Geometry check sheet. Reference: the model listing, model coordinates, mm. Face numbers are marked on the shaded views. Coordinates: 2 decimals unless noted, no trailing zeros. Write each loop counter-clockwise with the first axis right and the second up, starting at its lowest first coordinate (ties: lowest second). Pieces come first, ordered by that corner, then holes. Notation, with made-up numbers: (17, 44.25) -> (36, 44.25) arc R12 cw to (36, 48.25) -> close; hole circle Ø6 at (39.5, 71.25). An arc over 180 degrees is marked (long way). Answer in a Markdown table with one row per item. Add a question column.
1. Depth check by flat-ended pin: P1, Ø0.5, axis at x = 31.5, z = -72.5, coming from the +Y side; P2, Ø2.5, axis at x = -20.5, z = -49, coming from the +Y side; P3, Ø16.5, axis at x = 9, y = 7.5, coming from the -Z side. Enter the tip coordinate at first touch or a pass-through.
2. Mould release check, pull along Y, two halves, no side actions. Record for the marked faces 1, 2, 3 and 4: pulls with the +Y half, pulls with the -Y half, needs draft (parallel to the pull), parting line crosses it, or undercut.
3. Scan lines: L1, parallel to Y at x = 25, z = -16; L2, parallel to X at y = -13, z = -5.5; L3, parallel to X at y = 9.5, z = -63. Record each from-to range of solid material in increasing order. Write a range as from..to.
4. Cross-section at B-B on x = -20.5. Give the number of separate pieces and of enclosed holes in the cut face, and give its area (3 significant figures).
5. Cross-section at D-D on z = -66. Record the cut outline in (x, y).
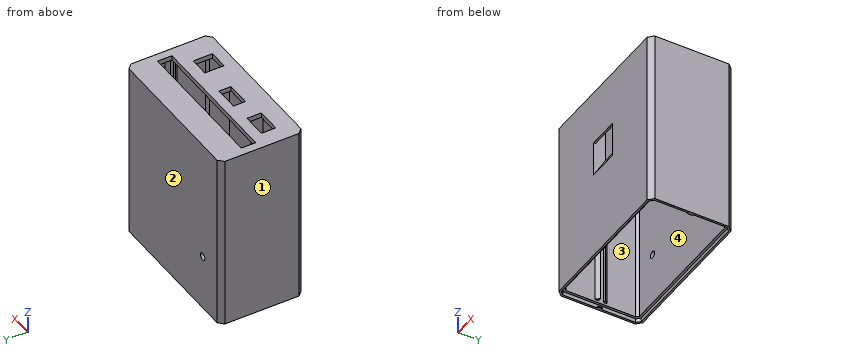
```python
from build123d import *
from OCP.BRepFilletAPI import BRepFilletAPI_MakeChamfer

# Parameters (mm, degrees)
CROQUIS1_W              = 3.5
CROQUIS1_H              = 6
CROQUIS1_W_2            = 10
CROQUIS1_H_2            = 5
CROQUIS1_W_3            = 8
CROQUIS1_H_3            = 8
SALIENTE_EXTRUIR1_DEPTH = 2
CROQUIS2_W              = 65
CROQUIS2_H              = 35
CROQUIS2_W_2            = 61
CROQUIS2_H_2            = 31
SALIENTE_EXTRUIR2_DEPTH = 71
SALIENTE_EXTRUIR3_DEPTH = 70
CORTAR_EXTRUIR2_REACH   = 87.57
CROQUIS9_R              = 1.5
CHAFL_N3_SIZE           = 2
CHAFL_N2_SIZE           = 1
BOSS_EXTRUDE1_DEPTH     = 1.5
CHAMFER1_SIZE           = 0.1
CHAMFER1_SIZE_2         = 1.5
SKETCH2_W               = 1
SKETCH2_H               = 2
BOSS_EXTRUDE2_DEPTH     = 0.5
SKETCH3_W               = 15
SKETCH3_H               = 20
BOSS_EXTRUDE3_DEPTH     = 7
SKETCH4_W               = 13
SKETCH4_H               = 18
CUT_EXTRUDE1_DEPTH      = 5
SKETCH5_W               = 13
SKETCH5_H               = 2.5
BOSS_EXTRUDE4_DEPTH     = 12
CHAMFER2_SIZE2          = 5
CHAMFER2_SIZE           = 8.660254038
CHAMFER3_SIZE2          = 5
CHAMFER3_SIZE           = 8.660254038
CHAMFER4_SIZE           = 3
CHAMFER4_SIZE2          = 1.732050808
BOSS_EXTRUDE5_REACH     = 76.315
SKETCH6_W               = 15
SKETCH6_H               = 5
BOSS_EXTRUDE6_REACH     = 171.868
SKETCH7_W               = 9.865861754
SKETCH7_H               = 0.5


with BuildPart() as part:
    # Croquis1 → Saliente-Extruir1 (new body)
    # profile 1 of 4: a face of its own
    with BuildSketch(Plane.XY):
        Polygon((-32.5, 6.5), (-29, 6.5), (29, 6.5), (32.5, 6.5), (32.5, 17.5), (-32.5, 17.5), align=None)
    # profile 2 of 4: a face of its own
    with BuildSketch(Plane.XY):
        with Locations((-30.75, 3.5)):
            Rectangle(CROQUIS1_W, CROQUIS1_H)
    # profile 3 of 4: a face of its own
    with BuildSketch(Plane.XY):
        with Locations((30.75, 3.5)):
            Rectangle(CROQUIS1_W, CROQUIS1_H)
    # profile 4 of 4: a face of its own
    with BuildSketch(Plane.XY):
        Polygon((29, 0.5), (-29, 0.5), (-32.5, 0.5), (-32.5, -17.5), (32.5, -17.5), (32.5, 0.5), align=None)
        with Locations((-20.5, -7)):
            Rectangle(CROQUIS1_W_2, CROQUIS1_H, mode=Mode.SUBTRACT)
        with Locations((-2, -6)):
            Rectangle(CROQUIS1_W_2, CROQUIS1_H_2, mode=Mode.SUBTRACT)
        with Locations((18.5, -8.5)):
            Rectangle(CROQUIS1_W_3, CROQUIS1_H_3, mode=Mode.SUBTRACT)
    extrude(amount=SALIENTE_EXTRUIR1_DEPTH)

    # Croquis2 → Saliente-Extruir2 (add)
    with BuildSketch(Plane(origin=(0, 0, 0), x_dir=(-1, 0, 0), z_dir=(0, 0, -1))):
        Rectangle(CROQUIS2_W, CROQUIS2_H)
        Rectangle(CROQUIS2_W_2, CROQUIS2_H_2, mode=Mode.SUBTRACT)
    extrude(amount=SALIENTE_EXTRUIR2_DEPTH)

    # Croquis3 → Saliente-Extruir3 (add)
    with BuildSketch(Plane(origin=(0, 0, 0), x_dir=(-1, 0, 0), z_dir=(0, 0, -1))):
        Polygon((-30.5, 1), (-29, 1), (-30.5, 2.5), align=None)
        Polygon((-30.5, -1), (-30.5, -2.5), (-29, -1), align=None)
        Polygon((30.5, -1), (29, -1), (30.5, -2.5), align=None)
        Polygon((30.5, 1), (30.5, 2.5), (29, 1), align=None)
    extrude(amount=SALIENTE_EXTRUIR3_DEPTH)

    # Croquis9 → Cortar-Extruir2 (cut, up to next)
    with BuildSketch(Plane(origin=(0, 17.5, 0), x_dir=(1, 0, 0), z_dir=(0, 1, 0)), mode=Mode.PRIVATE) as cortar_extruir2_sk1:
        with Locations(Location((-20.5, 49, 0), (0, 0, 270))):
            Circle(CROQUIS9_R)
    cortar_extruir2_tool1 = extrude(cortar_extruir2_sk1.sketch, amount=-CORTAR_EXTRUIR2_REACH, mode=Mode.PRIVATE) & part.part
    add(cortar_extruir2_tool1.solids().sort_by_distance((-20.5, 17.5, -49))[0], mode=Mode.SUBTRACT)

    # Chaflán3
    chafl_n3_edges = [part.edges().sort_by_distance(p)[0] for p in [
        (-32.5, -17.5, -34.5),
        (-32.5, 17.5, -34.5),
        (32.5, 17.5, -34.5),
        (32.5, -17.5, -34.5),
    ]]
    chamfer(chafl_n3_edges, length=CHAFL_N3_SIZE)

    # Chaflán2
    chafl_n2_edges = [part.edges().sort_by_distance(p)[0] for p in [
        (-30.5, 15.5, -35.5),
        (30.5, 15.5, -35.5),
        (30.5, -15.5, -35.5),
        (-30.5, -15.5, -35.5),
    ]]
    chamfer(chafl_n2_edges, length=CHAFL_N2_SIZE)

    # Sketch1 → Boss-Extrude1 (add)
    with BuildSketch(Plane(origin=(0, 0, -71), x_dir=(-1, 0, 0), z_dir=(0, 0, -1))):
        Polygon((-32.5, 15.5), (-32.5, -15.5), (-30.5, -17.5), (30.5, -17.5), (32.5, -15.5), (32.5, 15.5), (30.5, 17.5), (-30.5, 17.5), align=None)
        Polygon((-31.55, 15.106497116), (-31.55, -15.106497116), (-30.106497116, -16.55), (30.106497116, -16.55), (31.55, -15.106497116), (31.55, 15.106497116), (30.106497116, 16.55), (-30.106497116, 16.55), align=None, mode=Mode.SUBTRACT)
    extrude(amount=BOSS_EXTRUDE1_DEPTH)

    # Chamfer1
    chamfer1_edges_1 = [part.edges().sort_by_distance(p)[0] for p in [
        (0, -16.55, -72.5),
    ]]
    chamfer1_side_1 = [part.faces().sort_by_distance(p)[0] for p in [
        (0, -16.552, -72.5),
    ]]
    chamfer1_edges_2 = [part.edges().sort_by_distance(p)[0] for p in [
        (-30.828248558, -15.828248558, -72.5),
    ]]
    chamfer1_side_2 = [part.faces().sort_by_distance(p)[0] for p in [
        (-30.829662771, -15.829662771, -72.5),
    ]]
    chamfer1_edges_3 = [part.edges().sort_by_distance(p)[0] for p in [
        (-31.55, 0, -72.5),
    ]]
    chamfer1_side_3 = [part.faces().sort_by_distance(p)[0] for p in [
        (-31.552, 0, -72.5),
    ]]
    chamfer1_edges_4 = [part.edges().sort_by_distance(p)[0] for p in [
        (-30.828248558, 15.828248558, -72.5),
    ]]
    chamfer1_side_4 = [part.faces().sort_by_distance(p)[0] for p in [
        (-30.829662771, 15.829662771, -72.5),
    ]]
    chamfer1_edges_5 = [part.edges().sort_by_distance(p)[0] for p in [
        (0, 16.55, -72.5),
    ]]
    chamfer1_side_5 = [part.faces().sort_by_distance(p)[0] for p in [
        (0, 16.552, -72.5),
    ]]
    chamfer1_edges_6 = [part.edges().sort_by_distance(p)[0] for p in [
        (30.828248558, 15.828248558, -72.5),
    ]]
    chamfer1_side_6 = [part.faces().sort_by_distance(p)[0] for p in [
        (30.829662771, 15.829662771, -72.5),
    ]]
    chamfer1_edges_7 = [part.edges().sort_by_distance(p)[0] for p in [
        (31.55, 0, -72.5),
    ]]
    chamfer1_side_7 = [part.faces().sort_by_distance(p)[0] for p in [
        (31.552, 0, -72.5),
    ]]
    chamfer1_edges_8 = [part.edges().sort_by_distance(p)[0] for p in [
        (30.828248558, -15.828248558, -72.5),
    ]]
    chamfer1_side_8 = [part.faces().sort_by_distance(p)[0] for p in [
        (30.829662771, -15.829662771, -72.5),
    ]]
    chamfer1 = BRepFilletAPI_MakeChamfer(part.part.solid().wrapped)
    for e in chamfer1_edges_1:
        chamfer1.Add(CHAMFER1_SIZE - 0.0001, CHAMFER1_SIZE_2 - 0.0001, e.wrapped, chamfer1_side_1[0].wrapped)
    for e in chamfer1_edges_2:
        chamfer1.Add(CHAMFER1_SIZE - 0.0001, CHAMFER1_SIZE_2 - 0.0001, e.wrapped, chamfer1_side_2[0].wrapped)
    for e in chamfer1_edges_3:
        chamfer1.Add(CHAMFER1_SIZE - 0.0001, CHAMFER1_SIZE_2 - 0.0001, e.wrapped, chamfer1_side_3[0].wrapped)
    for e in chamfer1_edges_4:
        chamfer1.Add(CHAMFER1_SIZE - 0.0001, CHAMFER1_SIZE_2 - 0.0001, e.wrapped, chamfer1_side_4[0].wrapped)
    for e in chamfer1_edges_5:
        chamfer1.Add(CHAMFER1_SIZE - 0.0001, CHAMFER1_SIZE_2 - 0.0001, e.wrapped, chamfer1_side_5[0].wrapped)
    for e in chamfer1_edges_6:
        chamfer1.Add(CHAMFER1_SIZE - 0.0001, CHAMFER1_SIZE_2 - 0.0001, e.wrapped, chamfer1_side_6[0].wrapped)
    for e in chamfer1_edges_7:
        chamfer1.Add(CHAMFER1_SIZE - 0.0001, CHAMFER1_SIZE_2 - 0.0001, e.wrapped, chamfer1_side_7[0].wrapped)
    for e in chamfer1_edges_8:
        chamfer1.Add(CHAMFER1_SIZE - 0.0001, CHAMFER1_SIZE_2 - 0.0001, e.wrapped, chamfer1_side_8[0].wrapped)
    add(Compound.cast(chamfer1.Shape()), mode=Mode.REPLACE)  # a hair under: the kernel refuses the full size

    # Sketch2 → Boss-Extrude2 (add)
    with BuildSketch(Plane(origin=(0, 0, -72.5), x_dir=(-1, 0, 0), z_dir=(0, 0, -1))):
        with Locations((-31.65, 0)):
            Rectangle(SKETCH2_W, SKETCH2_H)
        with Locations((31.65, 0)):
            Rectangle(SKETCH2_W, SKETCH2_H)
    extrude(amount=-BOSS_EXTRUDE2_DEPTH)

    # Sketch3 → Boss-Extrude3 (add)
    with BuildSketch(Plane.XZ.offset(17.5)):
        with Locations((0, -18)):
            Rectangle(SKETCH3_W, SKETCH3_H)
    extrude(amount=-BOSS_EXTRUDE3_DEPTH)

    # Sketch4 → Cut-Extrude1 (cut)
    with BuildSketch(Plane.XZ.offset(17.5)):
        with Locations((0, -18)):
            Rectangle(SKETCH4_W, SKETCH4_H)
    extrude(amount=-CUT_EXTRUDE1_DEPTH, mode=Mode.SUBTRACT)

    # Sketch5 → Boss-Extrude4 (add)
    with BuildSketch(Plane(origin=(0, 0, -9), x_dir=(-1, 0, 0), z_dir=(0, 0, -1))):
        with Locations((0, -16.25)):
            Rectangle(SKETCH5_W, SKETCH5_H)
    extrude(amount=BOSS_EXTRUDE4_DEPTH)

    # Chamfer2
    chamfer2_edges = [part.edges().sort_by_distance(p)[0] for p in [
        (0, -15.5, -28),
    ]]
    chamfer2_side = [part.faces().sort_by_distance(p)[0] for p in [
        (0, -15.5, -28.1),
    ]]
    chamfer(chamfer2_edges, length=CHAMFER2_SIZE - 0.0001, length2=CHAMFER2_SIZE2 - 0.0001, reference=chamfer2_side[0])  # a hair under: the kernel refuses the full size

    # Chamfer3
    chamfer3_edges = [part.edges().sort_by_distance(p)[0] for p in [
        (0, -17.5, -27),
    ]]
    chamfer3_side = [part.faces().sort_by_distance(p)[0] for p in [
        (0, -17.5, -27.1),
    ]]
    chamfer(chamfer3_edges, length=CHAMFER3_SIZE - 0.0001, length2=CHAMFER3_SIZE2 - 0.0001, reference=chamfer3_side[0])  # a hair under: the kernel refuses the full size

    # Chamfer4
    chamfer4_edges = [part.edges().sort_by_distance(p)[0] for p in [
        (0, -15, -21),
    ]]
    chamfer4_side = [part.faces().sort_by_distance(p)[0] for p in [
        (0, -15, -15),
    ]]
    chamfer(chamfer4_edges, length=CHAMFER4_SIZE, length2=CHAMFER4_SIZE2, reference=chamfer4_side[0])

    # Sketch6 → Boss-Extrude5 (add, up to next)
    with BuildSketch(Plane.XY.offset(-8), mode=Mode.PRIVATE) as boss_extrude5_sk1:
        with Locations((0, -13)):
            Rectangle(SKETCH6_W, SKETCH6_H)
    boss_extrude5_tool1 = extrude(boss_extrude5_sk1.sketch, amount=BOSS_EXTRUDE5_REACH, mode=Mode.PRIVATE) - part.part
    add(boss_extrude5_tool1.solids().sort_by_distance((0, -13, -8))[0])

    # Boss-Extrude6: up to this plane
    boss_extrude6_end = Plane(origin=(-6.5, -12.5, -17), z_dir=(0, 0, 1))
    # Sketch7 → Boss-Extrude6 (add, up to the surface)
    with BuildSketch(Plane(origin=(0, -3.455771366, 1.995190528), x_dir=(1, 0, 0), z_dir=(0, 0.8660254037844395, -0.4999999999999988)), mode=Mode.PRIVATE) as boss_extrude6_sk1:
        with Locations((1.567069123, 22.838457268)):
            Rectangle(SKETCH7_W, SKETCH7_H)
    boss_extrude6_tool1 = split(extrude(boss_extrude6_sk1.sketch, amount=BOSS_EXTRUDE6_REACH, dir=(0, 0, 1), mode=Mode.PRIVATE), bisect_by=boss_extrude6_end, keep=Keep.BOTH, mode=Mode.PRIVATE)
    add(boss_extrude6_tool1.solids().sort_by_distance((1.567069, -14.875, -17.783494))[0])


solid = part.part
```
Results found:
| question | item | result |
|---|---|---|
| 1 | P1 | stops at y = 16.75 |
| 1 | P2 | stops at y = -15.5 |
| 1 | P3 | stops at z = -71 |
| 2 | face 1 | needs draft |
| 2 | face 2 | pulls with the +Y half |
| 2 | face 3 | undercut |
| 2 | face 4 | undercut |
| 3 | L1 | y = -17.5..-15.5, 15.5..17.5 |
| 3 | L2 | x = -32.5..-30.5, -7.5..7.5, 30.5..32.5 |
| 3 | L3 | x = -32.5..-30.5, 30.5..32.5 |
| 4 | separate pieces | 4 |
| 4 | enclosed holes | 0 |
| 4 | area | 327 mm^2 |
| 5 | outline | (-32.5, -15.5) -> (-30.5, -17.5) -> (30.5, -17.5) -> (32.5, -15.5) -> (32.5, 15.5) -> (30.5, 17.5) -> (-30.5, 17.5) -> (-32.5, 15.5) -> close; hole (-30.5, -14.5) -> (-29.5, -15.5) -> (29.5, -15.5) -> (30.5, -14.5) -> (30.5, -2.5) -> (29, -1) -> (30.5, -1) -> (30.5, 1) -> (29, 1) -> (30.5, 2.5) -> (30.5, 14.5) -> (29.5, 15.5) -> (-29.5, 15.5) -> (-30.5, 14.5) -> (-30.5, 2.5) -> (-29, 1) -> (-30.5, 1) -> (-30.5, -1) -> (-29, -1) -> (-30.5, -2.5) -> close |
